Can you work these out from the model? Positions are in its coordinate system, mm. A direction names the side the tool comes from. Coordinates: 2 decimals unless noted, no trailing zeros. Loops run counter-clockwise (first coordinate to the right, second up) from the corner with the lowest first, then second, coordinate; pieces in that order, holes last. Notation, with made-up numbers: M 73,6 L 127,6 A19 cw 127,43 Z; hole C -26,-16 d6. An arc over 180 degrees is marked long. Return JSON: item names as keys, results as strings. Group by question number.
```python
from build123d import *

# Parameters (mm, degrees)
SKETCH_2_R      = 2.25
EXTRUDE_1_DEPTH = 5
EXTRUDE_5_DEPTH = 100
EXTRUDE_START   = 100
EXTRUDE_7_DEPTH = 100


with BuildPart() as part:
    # 草图2 → 凸台-拉伸1 (new body)
    with BuildSketch(Plane(origin=(0, 0, 0), x_dir=(1, 0, 0), z_dir=(0, 1, 0))):
        Polygon((-11.75, 45), (-52.25, 45), (-52.25, -45), (52.25, -45), (52.25, 45), (11.75, 45), (11.75, 21), (-11.75, 21), align=None)
        with Locations(Location((-8, 16.75, 0), (0, 0, 270))):
            Circle(SKETCH_2_R, mode=Mode.SUBTRACT)
        with Locations(Location((-48, 40.75, 0), (0, 0, 270))):
            Circle(SKETCH_2_R, mode=Mode.SUBTRACT)
        with Locations(Location((-40, 40.75, 0), (0, 0, 270))):
            Circle(SKETCH_2_R, mode=Mode.SUBTRACT)
        with Locations(Location((-32, 40.75, 0), (0, 0, 270))):
            Circle(SKETCH_2_R, mode=Mode.SUBTRACT)
        with Locations(Location((-24, 40.75, 0), (0, 0, 270))):
            Circle(SKETCH_2_R, mode=Mode.SUBTRACT)
        with Locations(Location((-16, 40.75, 0), (0, 0, 270))):
            Circle(SKETCH_2_R, mode=Mode.SUBTRACT)
        with Locations(Location((0, 16.75, 0), (0, 0, 270))):
            Circle(SKETCH_2_R, mode=Mode.SUBTRACT)
        with Locations(Location((8, 16.75, 0), (0, 0, 270))):
            Circle(SKETCH_2_R, mode=Mode.SUBTRACT)
        with Locations(Location((16, 40.75, 0), (0, 0, 270))):
            Circle(SKETCH_2_R, mode=Mode.SUBTRACT)
        with Locations(Location((24, 40.75, 0), (0, 0, 270))):
            Circle(SKETCH_2_R, mode=Mode.SUBTRACT)
        with Locations(Location((32, 40.75, 0), (0, 0, 270))):
            Circle(SKETCH_2_R, mode=Mode.SUBTRACT)
        with Locations(Location((40, 40.75, 0), (0, 0, 270))):
            Circle(SKETCH_2_R, mode=Mode.SUBTRACT)
        with Locations(Location((48, 40.75, 0), (0, 0, 270))):
            Circle(SKETCH_2_R, mode=Mode.SUBTRACT)
    extrude(amount=EXTRUDE_1_DEPTH)

    # 草图7 → 凸台-拉伸5 (add)
    with BuildSketch(Plane(origin=(0, 5, 5), x_dir=(1, 0, 0), z_dir=(0, 1, 0))):
        with BuildLine():
            ThreePointArc((-29.462817643, -34.890487173), (-41.309546241, -29.634761226), (-52.25, -22.686804315))
            Line((-52.25, -22.686804315), (-52.25, -40))
            Line((-52.25, -40), (-34.57233047, -40))
            Line((-34.57233047, -40), (-29.462817643, -34.890487173))
        make_face()
        with BuildLine():
            ThreePointArc((52.25, -22.686804315), (41.309546241, -29.634761226), (29.462817643, -34.890487173))
            Line((29.462817643, -34.890487173), (34.57233047, -40))
            Line((34.57233047, -40), (52.25, -40))
            Line((52.25, -40), (52.25, -22.686804315))
        make_face()
    extrude(amount=EXTRUDE_5_DEPTH)

    # 草图7<5> → 凸台-拉伸7 (add)
    with BuildSketch(Plane(origin=(0, 5, 5), x_dir=(1, 0, 0), z_dir=(0, 1, 0)).offset(EXTRUDE_START)):
        with BuildLine():
            Line((52.25, -40), (52.25, -22.686804315))
            ThreePointArc((52.25, -22.686804315), (80.411596121, 13.000359287), (86.867715522, 58))
            Line((86.867715522, 58), (83.845095265, 58))
            ThreePointArc((83.845095265, 58), (0, -37), (-83.845095265, 58))
            Line((-83.845095265, 58), (-86.867715522, 58))
            ThreePointArc((-86.867715522, 58), (-80.411596121, 13.000359287), (-52.25, -22.686804315))
            Line((-52.25, -22.686804315), (-52.25, -40))
            Line((-52.25, -40), (-34.57233047, -40))
            Line((-34.57233047, -40), (-29.462817643, -34.890487173))
            ThreePointArc((-29.462817643, -34.890487173), (0, -40), (29.462817643, -34.890487173))
            Line((29.462817643, -34.890487173), (34.57233047, -40))
            Line((34.57233047, -40), (52.25, -40))
        make_face()
    extrude(amount=EXTRUDE_7_DEPTH)


solid = part.part
```
1) For faces 4 (the face through (-32.05, 103.6, 42.48)), 5 (the face through (-35, 94, 45)), 6 (the face through (-33, 105, 36)), which set-ups out of +Z, -Z, +X, -X, +Y, -Y let a thin tool reach every point of the face, with its end or its side?
2) Suppose I cut it at C-C, the plane z = 20. List the corners of the cut face in (x, y) for me, then the cut area to 3 significant figures.
3) Suppose I cut it at D-D, the plane y = 118. List the corners of the cut face in (x, z) for me, then the cut area to 3 significant figures.
4) Suppose I cut it at B-B, the plane z = -28.5. List the corners of the cut face in (x, y) for me.
5) Suppose I cut it at A-A, the plane y = 42. List the corners of the cut face in (x, z) for me, then the cut area to 3 significant figures.
6) If I drill on line 1 (X direction, y = 178.5, z = -42.5); line 2 (Y direction, x = 30, z = 29.5); line 3 (X direction, y = 188.5, z = -29.5), over which ranges is the centre line in solid material (lowest first)? Write a range as from..to.
7) For pin 1 (6 mm diameter, centred on x = 8, z = -16.75, fed in from +Y); pin 2 (4 mm diameter, centred on x = -40.5, y = 2, fed in from -Z); pin 3 (4 mm diameter, centred on y = 152.5, z = -13.5, fed in from -X); pin 4 (3.5 mm diameter, centred on x = -32, z = -40.75, fed in from -Y), each with a flat end and sliding along its axis, tell me the tip position at first contact or that it passes through.
8) If we mould it in two halves opening along Y, with no side actions, what happens to faces 1 (the face through (-7, 205, 43)), 2 (the face through (2.005, 154.3, 41.976)), 3 (the face through (41.47, 54.3, 34.55))? For each: +Y half, -Y half, draft (parallel to the pull), parting line (faces both ways), or undercut.
Returned:
{
 "1": {"face 4": "+Z, +Y", "face 5": "+Z, +X, -X, +Y, -Y", "face 6": "-Z"},
 "2": {"outline": "M -61.24,105 L -56.87,105 L -56.87,205 L -61.24,205 Z; M -52.25,0 L 52.25,0 L 52.25,5 L -52.25,5 Z; M 56.87,105 L 61.24,105 L 61.24,205 L 56.87,205 Z", "area": "1,400 mm²"},
 "3": {"outline": "M -86.87,-53 L -83.85,-53 A84.5 cw long 83.85,-53 L 86.87,-53 A87.5 ccw 52.25,27.69 L 52.25,45 L 34.57,45 L 29.46,39.89 A87.5 ccw -29.46,39.89 L -34.57,45 L -52.25,45 L -52.25,27.69 A87.5 ccw Z", "area": "1,330 mm²"},
 "4": {"outline": "M -86.37,105 L -83.33,105 L -83.33,205 L -86.37,205 Z; M -52.25,0 L -11.75,0 L -11.75,5 L -52.25,5 Z; M 11.75,0 L 52.25,0 L 52.25,5 L 11.75,5 Z; M 83.33,105 L 86.37,105 L 86.37,205 L 83.33,205 Z"},
 "5": {"outline": "M -52.25,27.69 A87.5 cw -29.46,39.89 L -34.57,45 L -52.25,45 Z; M 29.46,39.89 A87.5 cw 52.25,27.69 L 52.25,45 L 34.57,45 Z", "area": "452 mm²"},
 "6": {"line 1": "x = -87.5..-84.5, 84.5..87.5", "line 2": "y = 0..5", "line 3": "x = -86.53..-83.49, 83.49..86.53"},
 "7": {"pin 1": "stops at y = 5", "pin 2": "stops at z = -45", "pin 3": "stops at x = -83.23", "pin 4": "passes through"},
 "8": {"face 1": "+Y half", "face 2": "draft", "face 3": "undercut"}
}
